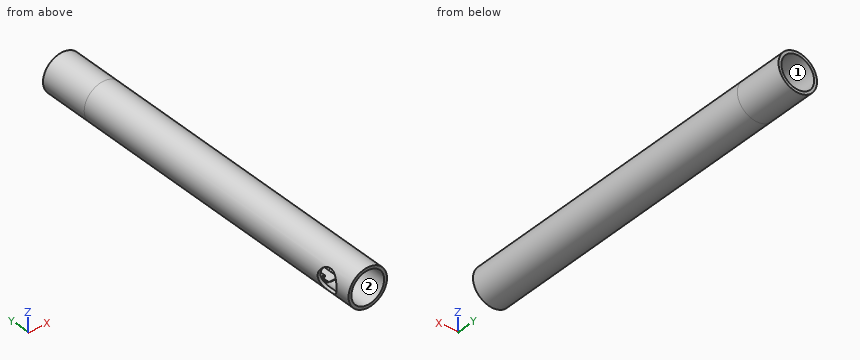
from build123d import *

# Parameters (mm, degrees)
F3_R      = 4.7
F4_DEPTH  = 67
F8_DEPTH  = 67
F6_R      = 4.7
F6_R_2    = 4
F9_DEPTH  = 10
F7_R      = 4.7
F7_R_2    = 4
F10_DEPTH = 12
F11_R     = 2.75
F12_DEPTH = 4.701


# Not quite as in the source:
# - ends of sketch curves that miss each other by under 0.0002 mm in the source are joined


with BuildPart() as f4:
    # F3 (on Front) → F4 (new body)
    with BuildSketch(Plane.XZ):
        Circle(F3_R)
    extrude(amount=F4_DEPTH)

    # F5 (on face) → F8 (cut, through all)
    with BuildSketch(Plane.XZ.offset(67)):
        with BuildLine():
            Line((-1.25, -3.8), (0, -3.8))
            Line((0, -3.8), (1.25, -3.8))
            Line((1.25, -3.8), (1.25, -3.7))
            ThreePointArc((1.25, -3.7), (1.3085786438, -3.5585786438), (1.45, -3.5))
            Line((1.45, -3.5), (2, -3.5))
            Line((2, -3.5), (2, -3.05))
            ThreePointArc((2, -3.05), (2.0585786438, -2.9085786438), (2.2, -2.85))
            Line((2.2, -2.85), (3.15, -2.85))
            Line((3.15, -2.85), (3.15, -2.15))
            Line((3.15, -2.15), (2.2, -2.15))
            ThreePointArc((2.2, -2.15), (2.0585786438, -2.0914213562), (2, -1.95))
            Line((2, -1.95), (2, -1.887459))
            ThreePointArc((2, -1.887459), (2.1033535752, -1.771554046), (2.2, -1.65))
            Line((2.2, -1.65), (3.75, -1.65))
            Line((3.75, -1.65), (3.75, 0))
            Line((3.75, 0), (3.75, 1.65))
            Line((3.75, 1.65), (2.2, 1.65))
            ThreePointArc((2.2, 1.65), (2.1033535752, 1.771554046), (1.9999998047, 1.8874588157))
            Line((1.9999998047, 1.8874588157), (2, 1.95))
            ThreePointArc((2, 1.95), (2.0585786438, 2.0914213562), (2.2, 2.15))
            Line((2.2, 2.15), (3.15, 2.15))
            Line((3.15, 2.15), (3.15, 2.85))
            Line((3.15, 2.85), (2.2, 2.85))
            ThreePointArc((2.2, 2.85), (2.0585786438, 2.9085786438), (2, 3.05))
            Line((2, 3.05), (2, 3.5))
            Line((2, 3.5), (1.45, 3.5))
            ThreePointArc((1.45, 3.5), (1.3085786438, 3.5585786438), (1.25, 3.7))
            Line((1.25, 3.7), (1.25, 3.8))
            Line((1.25, 3.8), (0, 3.8))
            Line((0, 3.8), (-1.25, 3.8))
            Line((-1.25, 3.8), (-1.25, 3.7))
            ThreePointArc((-1.25, 3.7), (-1.3085786438, 3.5585786438), (-1.45, 3.5))
            Line((-1.45, 3.5), (-2, 3.5))
            Line((-2, 3.5), (-2, 3.05))
            ThreePointArc((-2, 3.05), (-2.0585786438, 2.9085786438), (-2.2, 2.85))
            Line((-2.2, 2.85), (-3.15, 2.85))
            Line((-3.15, 2.85), (-3.15, 2.15))
            Line((-3.15, 2.15), (-2.2, 2.15))
            ThreePointArc((-2.2, 2.15), (-2.0585786438, 2.0914213562), (-2, 1.95))
            Line((-2, 1.95), (-2, 1.887459))
            ThreePointArc((-2, 1.887459), (-2.1033535752, 1.771554046), (-2.2, 1.65))
            Line((-2.2, 1.65), (-3.75, 1.65))
            Line((-3.75, 1.65), (-3.75, 0))
            Line((-3.75, 0), (-3.75, -1.65))
            Line((-3.75, -1.65), (-2.2, -1.65))
            ThreePointArc((-2.2, -1.65), (-2.1033535752, -1.771554046), (-1.9999998047, -1.8874588157))
            Line((-1.9999998047, -1.8874588157), (-2, -1.95))
            ThreePointArc((-2, -1.95), (-2.0585786438, -2.0914213562), (-2.2, -2.15))
            Line((-2.2, -2.15), (-3.15, -2.15))
            Line((-3.15, -2.15), (-3.15, -2.85))
            Line((-3.15, -2.85), (-2.2, -2.85))
            ThreePointArc((-2.2, -2.85), (-2.0585786438, -2.9085786438), (-2, -3.05))
            Line((-2, -3.05), (-2, -3.5))
            Line((-2, -3.5), (-1.45, -3.5))
            ThreePointArc((-1.45, -3.5), (-1.3085786438, -3.5585786438), (-1.25, -3.7))
            Line((-1.25, -3.7), (-1.25, -3.8))
        make_face()
    extrude(amount=-F8_DEPTH, mode=Mode.SUBTRACT)

    # F6 (on face) → F9 (join)
    with BuildSketch(Plane.XZ.offset(67)):
        Circle(F6_R)
        Circle(F6_R_2, mode=Mode.SUBTRACT)
    extrude(amount=F9_DEPTH)

    # F7 (on face) → F10 (join)
    with BuildSketch(Plane(origin=(0, 0, 0), x_dir=(-1, 0, 0), z_dir=(0, 1, 0))):
        Circle(F7_R)
        Circle(F7_R_2, mode=Mode.SUBTRACT)
    extrude(amount=F10_DEPTH)

    # F11 (on Right) → F12 (cut, through all)
    with BuildSketch(Plane.YZ):
        with Locations((-70.75, 0)):
            Circle(F11_R)
    extrude(amount=-F12_DEPTH, mode=Mode.SUBTRACT)


solid = f4.part
The listing builds one solid part. Answer for the finished solid, in the listing's coordinates (mm). Face numbers are marked on the shaded views. A direction names the side the tool comes from. Coordinates: 2 decimals unless noted, no trailing zeros. Order: outer loops, then holes, each group sorted by start corner. A loop starts at its lowest first (then second) coordinate and runs counter-clockwise, first axis right, second up. Notation, with made-up numbers: M -14.5,61.5 L -1.5,61.5 A18 cw -1.5,84.5 Z; hole C -16,27 d1. An arc over 180 degrees is marked long. Use CSV: the item, a comma, the result in double quotes.
Q1. Given pin 1 Ø1.5 at (y, z) = (-19, -2) entering from +X; pin 2 Ø4 at (x, z) = (1.5, -1) entering from +Y; pin 3 Ø5 at (x, y) = (3, -31.5) entering from +Z, each flat-ended and moving along its own axis, determine where each tip first touches the part or whether it passes through.
Here are the results:
pin 1,"x = 4.53"
pin 2,"y = 0"
pin 3,"z = 4.67"
Q2. Straight lines are drawn through the part: L1, parallel to Z at x = 3.5, y = -48.5; L2, parallel to Z at x = 0, y = -72.25; L3, parallel to Z at x = 3, y = -64.5. For each, find the intervals that lie inside material, in ascending order.
Here are the results:
L1,"-3.14 to -1.65, 1.65 to 3.14"
L2,"-4.7 to -4, 4 to 4.7"
L3,"-3.62 to -2.85, -2.15 to -1.65, 1.65 to 2.15, 2.85 to 3.62"
Q3. Section C-C (y = -70.75) is taken. Determine the outline of the cut face in (x, z), then the cut area to 3 significant figures.
Here are the results:
outline,"M -3.81,-2.75 A4.7 ccw long -3.81,2.75 L -2.9,2.75 A4 cw long -2.9,-2.75 Z"
area,"15.0 mm2"
Q4. Section B-B (z = 0) is taken. Determine the outline of the cut face in (x, y).
Here are the results:
outline,"M -4.7,-77 L -4,-77 L -4,-73.5 L -4.7,-73.5 Z; M -4.7,-68 L -4,-68 L -4,-67 L -3.75,-67 L -3.75,0 L -4,0 L -4,12 L -4.7,12 Z; M 3.75,-67 L 4,-67 L 4,-77 L 4.7,-77 L 4.7,12 L 4,12 L 4,0 L 3.75,0 Z"
Q5. Section A-A (x = 0) is taken. Determine the outline of the cut face in (y, z), then the cut area to 3 significant figures.
Here are the results:
outline,"M -77,-4.7 L 12,-4.7 L 12,-4 L 0,-4 L 0,-3.8 L -67,-3.8 L -67,-4 L -77,-4 Z; M -77,4 L -67,4 L -67,3.8 L 0,3.8 L 0,4 L 12,4 L 12,4.7 L -77,4.7 Z"
area,"151 mm2"
Q6. A tool of negligible diameter and unlimited length cuts with its end or side. For the marked faces 1 and 2, from which of +Z, -Z, +X, -X, +Y, -Y can it reach the whole face along a straight path? Write none if from no direction.
Here are the results:
face 1,"+Y"
face 2,"-Y"
